Here's how the part is built. I have some questions about the finished solid (model axes, mm). Round coordinates to 2 decimals unless told otherwise and drop trailing zeros. Write each loop counter-clockwise with the first axis right and the second up, starting at its lowest first coordinate (ties: lowest second). Pieces come first, ordered by that corner, then holes. Notation, with made-up numbers: (8, 35) - (55, 35) arc R23 cw to (55, 49) - close; hole circle Ø4 at (57, 35). An arc over 180 degrees is marked (long way). One line per item, written item: value. Start each with the question number.
Item 1: Imagine slicing it at A-A, the plane y = 0. Please give me the cut outline in (x, z), then the cut area to 3 significant figures.
Item 2: Imagine slicing it at D-D, the plane z = 4.25. Please give me the cut outline in (x, y), then the cut area to 3 significant figures.
Item 3: Imagine slicing it at B-B, the plane x = 2. Please give me the cut outline in (y, z), then the cut area to 3 significant figures.
Item 4: If I drill on line 1 (Z direction, x = 1.8, y = 0); line 2 (Y direction, x = 1.4, z = -0.75); line 3 (Z direction, x = 1, y = 1), over which ranges is the centre line in solid material (lowest first)?
Item 5: Thinking about a two-plate mould opening in Z: for faces 1 (the face through (1, 0, -5)), 2 (the face through (1.232, -4.31, 2.535)), 3 (the face through (1.23, -0.54, -2.44)), which applies, released by +Z, released by -Z, zero draft, split by the parting line, or undercut?
Item 6: For P1, Ø1.5, axis at x = 2, y = 3, coming from the -Z side, with a flat end and sliding along its axis, tell me the tip position at first contact or that it passes through.
Item 7: Imagine slicing it at C-C, the plane z = 0.75. Please give me the cut outline in (x, y), then the cut area to 3 significant figures.
```python
from build123d import *

# Parameters (mm, degrees)
F0_R     = 2.5
F1_DEPTH = 2.5


with BuildPart() as f1:
    # F0 (on Right) → F1 (new body)
    with BuildSketch(Plane.YZ):
        Polygon((2.886751, 5), (-2.886751, 5), (-5.773503, 0), (-2.886751, -5), (2.886751, -5), (5.773503, 0), align=None)
        Circle(F0_R, mode=Mode.SUBTRACT)
    extrude(amount=F1_DEPTH)


solid = f1.part
```
Values follow:
1. outline: (0, -5) - (2.5, -5) - (2.5, -2.5) - (0, -2.5) - close; (0, 2.5) - (2.5, 2.5) - (2.5, 5) - (0, 5) - close
1. area: 12.5 mm^2
2. outline: (0, -3.32) - (2.5, -3.32) - (2.5, 3.32) - (0, 3.32) - close
2. area: 16.6 mm^2
3. outline: (-5.77, 0) - (-2.89, -5) - (2.89, -5) - (5.77, 0) - (2.89, 5) - (-2.89, 5) - close; hole circle Ø5 at (0, 0)
3. area: 67.0 mm^2
4. line 1: z = -5 to -2.5, 2.5 to 5
4. line 2: y = -5.34 to -2.38, 2.38 to 5.34
4. line 3: z = -5 to -2.29, 2.29 to 5
5. face 1: released by -Z
5. face 2: released by +Z
5. face 3: undercut
6. P1: stops at z = -5
7. outline: (0, -5.34) - (2.5, -5.34) - (2.5, -2.38) - (0, -2.38) - close; (0, 2.38) - (2.5, 2.38) - (2.5, 5.34) - (0, 5.34) - close
7. area: 14.8 mm^2
